Build history of the part. All positions in model axes, mm. A direction names the side the tool comes from. Coordinates: 2 decimals unless noted, no trailing zeros. Loops run counter-clockwise (first coordinate to the right, second up) from the corner with the lowest first, then second, coordinate; pieces in that order, holes last. Notation, with made-up numbers: (62, 49) -> (66, 49) arc R34 cw to (66, 81) -> close; hole circle Ø8 at (35, 74). An arc over 180 degrees is marked (long way). One line per item, written item: value. Start each with the question number.
```python
from build123d import *

# Parameters (mm, degrees)
ESQUISSE1_W             = 24.75
ESQUISSE1_H             = 14.45
BOSS_EXTRU_1_DEPTH      = 0.8
ESQUISSE2_W             = 5
ESQUISSE2_H             = 5
BOSS_EXTRU_2_DEPTH      = 0.95
ESQUISSE4_W             = 4.1
ESQUISSE4_H             = 5.1
BOSS_EXTRU_3_DEPTH      = 1.6
ESQUISSE5_R             = 0.8
ENL_V_MAT_EXTRU_1_DEPTH = 1.6
ENL_V_MAT_EXTRU_2_DEPTH = 0.01


with BuildPart() as part:
    # Esquisse1 → Boss.-Extru.1 (new body)
    with BuildSketch(Plane(origin=(0, 0, 0), x_dir=(1, 0, 0), z_dir=(0, 1, 0))):
        Rectangle(ESQUISSE1_W, ESQUISSE1_H)
    extrude(amount=BOSS_EXTRU_1_DEPTH)

    # Esquisse2 → Boss.-Extru.2 (add)
    with BuildSketch(Plane(origin=(0, 0.8, 0), x_dir=(1, 0, 0), z_dir=(0, 1, 0))):
        with Locations((-1.875, 2.425)):
            Rectangle(ESQUISSE2_W, ESQUISSE2_H)
    extrude(amount=BOSS_EXTRU_2_DEPTH)

    # Esquisse4 → Boss.-Extru.3 (add)
    with BuildSketch(Plane(origin=(0, 0.8, 0), x_dir=(1, 0, 0), z_dir=(0, 1, 0))):
        with Locations((-1.875, -3.975)):
            Rectangle(ESQUISSE4_W, ESQUISSE4_H)
    extrude(amount=BOSS_EXTRU_3_DEPTH)

    # Esquisse5 → Enlèv. mat.-Extru.1 (cut)
    with BuildSketch(Plane(origin=(0, 0.8, 0), x_dir=(1, 0, 0), z_dir=(0, 1, 0))):
        with Locations(Location((-10.875, -4.125, 0), (0, 0, 270))):
            Circle(ESQUISSE5_R)
        with Locations(Location((-10.875, -1.375, 0), (0, 0, 270))):
            Circle(ESQUISSE5_R)
        with Locations(Location((-10.875, 1.375, 0), (0, 0, 270))):
            Circle(ESQUISSE5_R)
        with Locations(Location((-10.875, 4.125, 0), (0, 0, 270))):
            Circle(ESQUISSE5_R)
        with Locations(Location((-8.175, 4.125, 0), (0, 0, 270))):
            Circle(ESQUISSE5_R)
        with Locations(Location((-8.175, 1.375, 0), (0, 0, 270))):
            Circle(ESQUISSE5_R)
        with Locations(Location((-8.175, -1.375, 0), (0, 0, 270))):
            Circle(ESQUISSE5_R)
        with Locations(Location((-8.175, -4.125, 0), (0, 0, 270))):
            Circle(ESQUISSE5_R)
    extrude(amount=-ENL_V_MAT_EXTRU_1_DEPTH, mode=Mode.SUBTRACT)

    # Esquisse6 → Enlèv. mat.-Extru.2 (cut)
    with BuildSketch(Plane(origin=(0, 0.8, 0), x_dir=(1, 0, 0), z_dir=(0, 1, 0))):
        Polygon((3.875, 5.625), (11.775, 5.625), (11.775, 3.925), (8.075, 3.925), (8.075, 3.258333333), (11.775, 3.258333333), (11.775, 1.558333333), (8.075, 1.558333333), (8.075, 0.891666667), (11.775, 0.891666667), (11.775, -0.808333333), (8.075, -0.808333333), (8.075, -1.475), (11.775, -1.475), (11.775, -5.975), (11.175, -5.975), (11.175, -2.075), (7.475, -2.075), (7.475, -0.208333333), (11.175, -0.208333333), (11.175, 0.291666667), (7.475, 0.291666667), (7.475, 2.158333333), (11.175, 2.158333333), (11.175, 2.658333333), (7.475, 2.658333333), (7.475, 4.525), (11.175, 4.525), (11.175, 5.025), (5.075, 5.025), (5.075, -2.075), (4.475, -2.075), (4.475, 5.025), (3.875, 5.025), align=None)
    extrude(amount=-ENL_V_MAT_EXTRU_2_DEPTH, mode=Mode.SUBTRACT)


solid = part.part
```
Item 1: Tool access for faces 5 (the face through (-4.375, 1, -2)), 6 (the face through (-3.925, 2, 4)), 7 (the face through (-2, 1, 0.075)), 8 (the face through (-2, 1.75, -2)): list every direction of +Z, -Z, +X, -X, +Y, -Y with a clear straight run to the whole face (end or side of a thin tool).
Item 2: Band-saw the part on A-A, the plane y = 1.2. List the corners of the cut face in (x, z) (3 decimals), and give its area (3 significant figures).
Item 3: Probe probe 1 along Z at (x, y) = (-10.25, 0.3) (3 decimals); probe 2 along X at (y, z) = (0.65, 4.5) (3 decimals); probe 3 along Y at (x, z) = (2, -4.25). List the from-to ranges inside material, lowest first.
Item 4: Two-plate mould, pull along Z, no slides. Class faces 1 (the face through (0, 0, 0)), 2 (the face through (-8.956, 0.406, 1.202)), 3 (the face through (-2, 2, 6.525)), 4 (the face through (-8.66, 0.41, 3.49)): +Z half, -Z half, draft (parallel to the pull), parting line (faces both ways), or undercut.
Item 5: Drop flat-ended pins along their axis: pin 1 Ø6 at (x, z) = (-7.5, 5) entering from +Y; pin 2 Ø4 at (x, z) = (-2, -1) entering from +Y; pin 3 Ø0.5 at (y, z) = (1.5, -2) entering from +X (3 decimals). Give the stop position or say it passes through.
Item 6: Band-saw the part on D-D, the plane z = 5.25. List the corners of the cut face in (x, y) (3 decimals).
Item 7: Band-saw the part on C-C, the plane x = -0.75. List the corners of the cut face in (y, z) (3 decimals), and give its area (3 significant figures).
Item 8: Band-saw the part on B-B, the plane z = -4.25. List the corners of the cut face in (x, y) (3 decimals), and give its area (3 significant figures).
Worked out:
1. face 5: +Z, -Z, -X, +Y
1. face 6: +Z, -X, +Y
1. face 7: +X, -X, +Y
1. face 8: -Z, +X, -X, +Y
2. outline: (-4.375, -4.925) -> (0.625, -4.925) -> (0.625, 0.075) -> (-4.375, 0.075) -> close; (-3.925, 1.425) -> (0.175, 1.425) -> (0.175, 6.525) -> (-3.925, 6.525) -> close
2. area: 45.9 mm²
3. probe 1: z = -7.225 to -4.624, -3.626 to -1.874, -0.876 to 0.876, 1.874 to 3.626, 4.624 to 7.225
3. probe 2: x = -12.375 to -11.582, -10.168 to -8.882, -7.468 to 12.375
3. probe 3: y = 0 to 0.8
4. face 1: draft
4. face 2: undercut
4. face 3: +Z half
4. face 4: undercut
5. pin 1: stops at y = 0.8
5. pin 2: stops at y = 1.75
5. pin 3: stops at x = 0.625
6. outline: (-12.375, 0) -> (12.375, 0) -> (12.375, 0.8) -> (11.775, 0.8) -> (11.775, 0.79) -> (11.175, 0.79) -> (11.175, 0.8) -> (0.175, 0.8) -> (0.175, 2.4) -> (-3.925, 2.4) -> (-3.925, 0.8) -> (-12.375, 0.8) -> close
7. outline: (0, -7.225) -> (0.8, -7.225) -> (0.8, -4.925) -> (1.75, -4.925) -> (1.75, 0.075) -> (0.8, 0.075) -> (0.8, 1.425) -> (2.4, 1.425) -> (2.4, 6.525) -> (0.8, 6.525) -> (0.8, 7.225) -> (0, 7.225) -> close
7. area: 24.5 mm²
8. outline: (-12.375, 0) -> (-11.665, 0) -> (-11.665, 0.8) -> (-12.375, 0.8) -> close; (-10.085, 0) -> (-8.965, 0) -> (-8.965, 0.8) -> (-10.085, 0.8) -> close; (-7.385, 0) -> (12.375, 0) -> (12.375, 0.8) -> (11.775, 0.8) -> (11.775, 0.79) -> (7.475, 0.79) -> (7.475, 0.8) -> (5.075, 0.8) -> (5.075, 0.79) -> (4.475, 0.79) -> (4.475, 0.8) -> (0.625, 0.8) -> (0.625, 1.75) -> (-4.375, 1.75) -> (-4.375, 0.8) -> (-7.385, 0.8) -> close
8. area: 22.0 mm²
